Verification items for this drawing (mm, ordinates from the low corner). A direction names the side the tool comes from. Round coordinates to 2 decimals unless told otherwise and drop trailing zeros. Write each loop counter-clockwise with the first axis right and the second up, starting at its lowest first coordinate (ties: lowest second). Pieces come first, ordered by that corner, then holes. Notation, with made-up numbers: (30.25, 75.25) -> (61.25, 75.25) arc R23 ccw to (61.25, 110.25) -> close; hole circle Ø5 at (0.25, 19). An arc over 180 degrees is marked (long way). One line per item, written item: value.
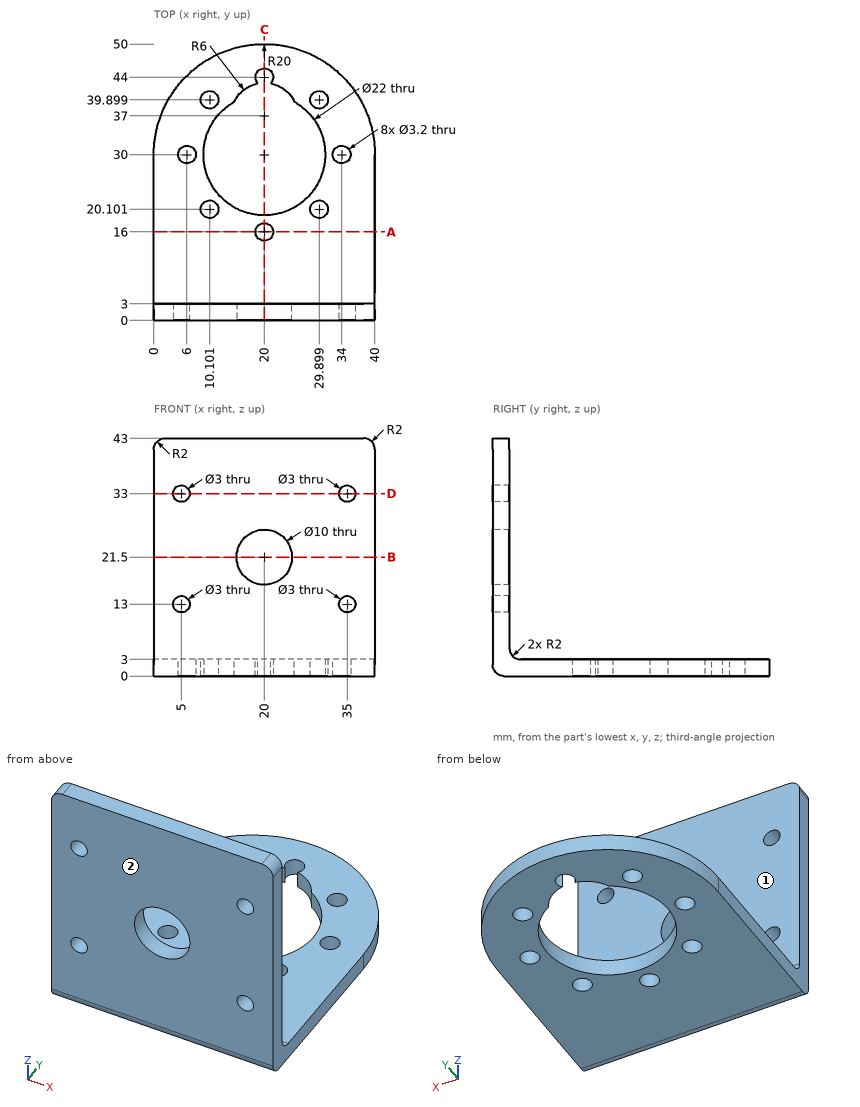
Item 1: Tool access check on the marked faces 1 and 2. Record the directions out of +Z, -Z, +X, -X, +Y, -Y that give a thin tool (end or side, any length) a straight path to the whole face; none if there is none.
Result set:
face 1: +Z, +X, -X, +Y
face 2: +Z, -Z, +X, -X, -Y
Item 2: Sectioned sample at D-D (z = 33). Enter the section's corners in (x, y), then the cut area to 3 significant figures.
Result set:
outline: (0, 0) -> (3.5, 0) -> (3.5, 3) -> (0, 3) -> close; (6.5, 0) -> (33.5, 0) -> (33.5, 3) -> (6.5, 3) -> close; (36.5, 0) -> (40, 0) -> (40, 3) -> (36.5, 3) -> close
area: 102 mm^2
Item 3: Depth check by flat-ended pin: pin 1 (8 mm diameter, centred on x = 7, y = 27.5, fed in from +Z); pin 2 (5 mm diameter, centred on x = 5, z = 33, fed in from +Y); pin 3 (3 mm diameter, centred on x = 14.5, y = 23.5, fed in from -Z); pin 4 (10 mm diameter, centred on x = 20, z = 18, fed in from -Y). Enter the tip coordinate at first touch or a pass-through.
Result set:
pin 1: z = 3
pin 2: y = 3
pin 3: through
pin 4: y = 0
Item 4: Sectioned sample at B-B (z = 21.5). Enter the section's corners in (x, y).
Result set:
outline: (0, 0) -> (15, 0) -> (15, 3) -> (0, 3) -> close; (25, 0) -> (40, 0) -> (40, 3) -> (25, 3) -> close
Item 5: Sectioned sample at C-C (x = 20). Enter the section's corners in (y, z).
Result set:
outline: (0, 2) arc R2 ccw to (2, 0) -> (14.4, 0) -> (14.4, 3) -> (5, 3) arc R2 cw to (3, 5) -> (3, 16.5) -> (0, 16.5) -> close; (0, 26.5) -> (3, 26.5) -> (3, 43) -> (0, 43) -> close; (17.6, 0) -> (19, 0) -> (19, 3) -> (17.6, 3) -> close; (45.6, 0) -> (50, 0) -> (50, 3) -> (45.6, 3) -> close
Item 6: Sectioned sample at A-A (y = 16). Enter the section's corners in (x, z).
Result set:
outline: (0, 0) -> (18.4, 0) -> (18.4, 3) -> (0, 3) -> close; (21.6, 0) -> (40, 0) -> (40, 3) -> (21.6, 3) -> close
Item 7: Material ranges on line 1 along Z through (x, y) = (35, 1.75) (1 decimal); line 2 along Z through (x, y) = (27, 15), recorded low to high.
Result set:
line 1: 0 to 11.5, 14.5 to 31.5, 34.5 to 43
line 2: 0 to 3
